The listing builds one solid part. Answer for the finished solid, in the listing's coordinates (mm). Round coordinates to 2 decimals unless told otherwise and drop trailing zeros. Order: outer loops, then holes, each group sorted by start corner. A loop starts at its lowest first (then second) coordinate and runs counter-clockwise, first axis right, second up. Notation, with made-up numbers: (-18, -21.5) - (27, -21.5) arc R35 cw to (27, 15.5) - close; hole circle Ø4 at (82.25, 33). An arc over 180 degrees is marked (long way). One line per item, written item: value. Start each with the question number.
1. Straight lines are drawn through the part: line 1 (Y direction, x = 0.3, z = 753); line 2 (X direction, y = 16.75, z = 622) (3 decimals); line 3 (Y direction, x = 2.7, z = 252). For each, find the intervals that lie inside material, in ascending order.
2. Section A-A, the plane z = 139 is taken. Give the vertices of the cut face in (x, y) (3 decimals).
3. Flat-ended cylindrical pins translate along their axes: P1, Ø2, axis at x = 4, y = 9.5, coming from the +Z side; P2, Ø1, axis at x = 3, z = 544.5, coming from the -Y side. Find the tip coordinate at first contact, or state that the pin passes through.
from build123d import *

# Parameters (mm, degrees)
BOSS_EXTRUDE1_DEPTH = 1000
FILLET1_R           = 0.50329666
FILLET2_R           = 0.50398302
FILLET3_R           = 0.30157619
FILLET4_R           = 0.30157551
CUT_EXTRUDE1_DEPTH  = 2.375
LPATTERN1_COUNT     = 20
LPATTERN1_PITCH     = 50


with BuildPart() as part:
    # Sketch1 → Boss-Extrude1 (new body)
    with BuildSketch(Plane.XY):
        with BuildLine():
            Line((0, 20.330194912), (2.019589054, 22.349783966))
            ThreePointArc((2.019589054, 22.349783966), (2.375, 22.497), (2.730410946, 22.349783966))
            Line((2.730410946, 22.349783966), (4.75, 20.330194912))
            Line((4.75, 20.330194912), (4.75, 19.5291))
            Line((4.75, 19.5291), (2.375, 19.5291))
            Line((2.375, 19.5291), (2.375, 0))
            Line((2.375, 0), (0, 0))
            Line((0, 0), (0, 20.330194912))
        make_face()
    extrude(amount=BOSS_EXTRUDE1_DEPTH)

    # Fillet1
    fillet1_edges = [part.edges().sort_by_distance(p)[0] for p in [
        (0, 20.330194912, 500),
    ]]
    fillet(fillet1_edges, radius=FILLET1_R)

    # Fillet2
    fillet2_edges = [part.edges().sort_by_distance(p)[0] for p in [
        (4.75, 20.330194912, 500),
    ]]
    fillet(fillet2_edges, radius=FILLET2_R)

    # Fillet3
    fillet3_edges = [part.edges().sort_by_distance(p)[0] for p in [
        (4.75, 19.5291, 500),
    ]]
    fillet(fillet3_edges, radius=FILLET3_R)

    # Fillet4
    fillet4_edges = [part.edges().sort_by_distance(p)[0] for p in [
        (2.375, 0, 500),
        (0, 0, 500),
    ]]
    fillet(fillet4_edges, radius=FILLET4_R)

    # Sketch2 → Cut-Extrude1 (cut)
    with BuildSketch(Plane.ZY):
        with BuildLine():
            Line((27.65, 13.1043), (27.65, 6.4043))
            ThreePointArc((27.65, 6.4043), (25, 3.7543), (22.35, 6.4043))
            Line((22.35, 6.4043), (22.35, 13.1043))
            ThreePointArc((22.35, 13.1043), (25, 15.7543), (27.65, 13.1043))
        make_face()
    cut_extrude1 = extrude(amount=-CUT_EXTRUDE1_DEPTH, mode=Mode.SUBTRACT)

    # LPattern1: Cut-Extrude1 ×20
    with Locations(*[(0, 0, i * LPATTERN1_PITCH) for i in range(1, LPATTERN1_COUNT)]):
        add(cut_extrude1, mode=Mode.SUBTRACT)


solid = part.part
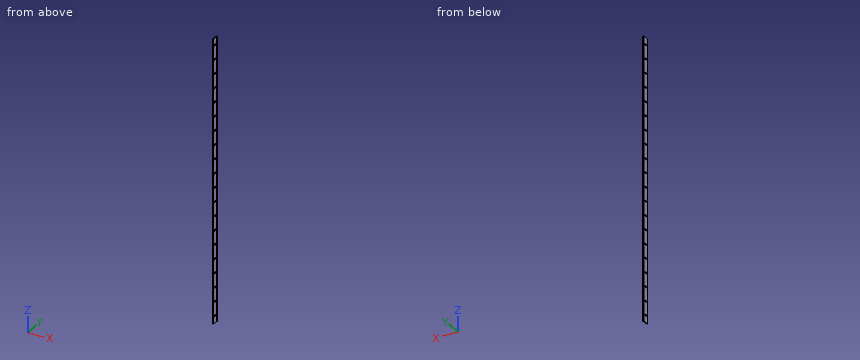
Answer list:
1. line 1: y = 0 to 20.63
1. line 2: x = 0 to 2.375
1. line 3: y = 19.53 to 22.38
2. outline: (0, 0.302) arc R0.302 ccw to (0.302, 0) - (2.073, 0) arc R0.302 ccw to (2.375, 0.302) - (2.375, 19.529) - (4.448, 19.529) arc R0.302 ccw to (4.75, 19.831) - (4.75, 20.121) arc R0.504 ccw to (4.602, 20.478) - (2.73, 22.35) arc R0.503 ccw to (2.02, 22.35) - (0.147, 20.478) arc R0.503 ccw to (0, 20.122) - close
3. P1: passes through
3. P2: stops at y = 19.53
